Input: part model. Units: mm. Frame: model coordinates. Give positions to 0.01 mm unless a question says otherwise; leave off trailing zeros. Order: outer loops, then holes, each group sorted by start corner. A loop starts at its lowest first (then second) coordinate and runs counter-clockwise, first axis right, second up. Notation, with made-up numbers: (75.25, 76) - (99.25, 76) arc R24 ccw to (99.25, 112) - close; hole circle Ø10 at (64.25, 42.25). An arc over 180 degrees is marked (long way). Answer in a Markdown table with one row per item. Add a question column.
1. Ray query, line 1 (Z direction, x = -46.5, y = -1.6); line 2 (X direction, y = -0.2, z = -20.5); line 3 (Z direction, x = 63, y = 0.45). Return the intervals inside material, ascending. Write a range as [from, to].
2. Section query B-B on z = -58. Return loops of the section in (x, y), and give its area (3 significant figures).
3. Mould query, pull axis Z, two halves, no side actions, for faces 1 (the face through (-17, -2.5, -1)), 2 (the face through (-55.55, 0.035, 42.594)), 3 (the face through (-11.99, -0.04, -0.53)). Classes: released by +Z, released by -Z, zero draft, split by the parting line, or undercut.
4. Section query C-C on x = 34.5. Return loops of the section in (y, z), and give its area (3 significant figures).
5. Section query A-A on y = -0.1. Count the separate pieces of the cut face and the enclosed holes in it, and give its area (3 significant figures).
6. Contact query for flat-ended pins moving along their axis: pin 1 (2.5 mm diameter, centred on x = -46, z = 0, fed in from -Y); pin 2 (2 mm diameter, centred on x = -0.5, y = 0, fed in from -Z); pin 3 (1 mm diameter, centred on y = 0.5, z = 2.5, fed in from +X). Output: stop coordinate, or through.
```python
from build123d import *

# Parameters (mm, degrees)
SKETCH_1_R      = 70
SKETCH_1_R_2    = 1.45
SKETCH_1_R_3    = 12
EXTRUDE_1_DEPTH = 2.5


with BuildPart() as part:
    # 草图1 → 凸台-拉伸1 (new body, symmetric)
    with BuildSketch(Plane(origin=(0, 0, 0), x_dir=(1, 0, 0), z_dir=(0, 1, 0))):
        Circle(SKETCH_1_R)
        with Locations((7.954951288, 20.329319959)):
            Circle(SKETCH_1_R_2, mode=Mode.SUBTRACT)
        with Locations((20.329319959, 7.954951288)):
            Circle(SKETCH_1_R_2, mode=Mode.SUBTRACT)
        Circle(SKETCH_1_R_3, mode=Mode.SUBTRACT)
        with Locations((30, 0)):
            Circle(SKETCH_1_R_2, mode=Mode.SUBTRACT)
        with Locations((46, 0)):
            Circle(SKETCH_1_R_2, mode=Mode.SUBTRACT)
        with Locations((62, 0)):
            Circle(SKETCH_1_R_2, mode=Mode.SUBTRACT)
        with Locations((0, 30)):
            Circle(SKETCH_1_R_2, mode=Mode.SUBTRACT)
        with Locations((0, 46)):
            Circle(SKETCH_1_R_2, mode=Mode.SUBTRACT)
        with Locations((0, 62)):
            Circle(SKETCH_1_R_2, mode=Mode.SUBTRACT)
        with Locations((-30, 0)):
            Circle(SKETCH_1_R_2, mode=Mode.SUBTRACT)
        with Locations((-46, 0)):
            Circle(SKETCH_1_R_2, mode=Mode.SUBTRACT)
        with Locations((-62, 0)):
            Circle(SKETCH_1_R_2, mode=Mode.SUBTRACT)
        with Locations((0, -30)):
            Circle(SKETCH_1_R_2, mode=Mode.SUBTRACT)
        with Locations((0, -46)):
            Circle(SKETCH_1_R_2, mode=Mode.SUBTRACT)
        with Locations((0, -62)):
            Circle(SKETCH_1_R_2, mode=Mode.SUBTRACT)
    extrude(amount=EXTRUDE_1_DEPTH, both=True)


solid = part.part
```
Answer:
| question | item | result |
|---|---|---|
| 1 | line 1 | z = [-52.32, -1.36], [1.36, 52.32] |
| 1 | line 2 | x = [-66.93, 6.52], [9.39, 66.93] |
| 1 | line 3 | z = [-30.51, -1.05], [1.05, 30.51] |
| 2 | outline | (-39.19, -2.5) - (39.19, -2.5) - (39.19, 2.5) - (-39.19, 2.5) - close |
| 2 | area | 392 mm² |
| 3 | face 1 | zero draft |
| 3 | face 2 | split by the parting line |
| 3 | face 3 | undercut |
| 4 | outline | (-2.5, -60.91) - (2.5, -60.91) - (2.5, 60.91) - (-2.5, 60.91) - close |
| 4 | area | 609 mm² |
| 5 | separate pieces | 1 |
| 5 | enclosed holes | 15 |
| 5 | area | 14,800 mm² |
| 6 | pin 1 | passes through |
| 6 | pin 2 | stops at z = -70 |
| 6 | pin 3 | stops at x = 69.97 |
